CAD build for the part. Positions are in the model's coordinates, mm. Give positions to 0.01 mm unless a question says otherwise; leave off trailing zeros. Write each loop counter-clockwise with the first axis right and the second up, starting at its lowest first coordinate (ties: lowest second). Pieces come first, ordered by that corner, then holes. Notation, with made-up numbers: (-30.75, 14) - (21.25, 14) arc R17 ccw to (21.25, 39) - close; hole circle Ø3 at (51, 29.25). An arc over 180 degrees is marked (long way). Put each result on its own line as item: value. Start each with the question number.
1. Mould opens along X. For faces 1 (the flat face through (-34, 0, 33)), 2 (the cylindrical face through (-10.84, 98.6, 48.81)), 3 (the cylindrical face through (-10.189, 98.6, 45.882)) say: +X half, -X half, draft (parallel to the pull), parting line (faces both ways), or undercut.
2. Wall check: line 1 (Z direction, x = 0, y = 80.5); line 2 (X direction, y = 63, z = 24). Give the ranges that are in metal, low to high.
3. Drop flat-ended pins along their axis: pin 1 (1 mm diameter, centred on y = 99.5, z = 15, fed in from +X); pin 2 (6 mm diameter, centred on x = -35, y = 69.5, fed in from +Z); pin 3 (8 mm diameter, centred on y = 81, z = 32, fed in from +X). Give the stop position or say it passes through.
4. Cut at C-C on y = 52. List the corners of the cut face in (x, z).
5. Cut at B-B on x = 0. List the corners of the cut face in (y, z).
6. Cut at A-A on z = 0. List the corners of the cut face in (x, y), and give its area (3 significant figures).
from build123d import *

# Parameters (mm, degrees)
EXTRUDE_1_OUTLINE_R      = 50
EXTRUDE_1_OUTLINE_R_2    = 47
EXTRUDE_1_DEPTH          = 200
CUT_EXTRUDE_1_DEPTH      = 213.132034356
CUT_EXTRUDE_1_DEPTH_BACK = 213.132034356
SKETCH_2_R               = 62.5


# Read off the part's stored shape, not the designer's step: Вытянуть-Тонкостенный1
with BuildPart() as part:
    # Вытянуть-Тонкостенный1 outline → Вытянуть-Тонкостенный1 (new body)
    with BuildSketch(Plane(origin=(0, 0, 0), x_dir=(1, 0, 0), z_dir=(0, 1, 0))):
        Circle(EXTRUDE_1_OUTLINE_R)
        Circle(EXTRUDE_1_OUTLINE_R_2, mode=Mode.SUBTRACT)
    extrude(amount=EXTRUDE_1_DEPTH)

    # Эскиз2 → Вырез-Вытянуть1 (cut, two sides: drawn at the far end of the back side and taken through both)
    with BuildSketch(Plane(origin=(0, 0, 0), x_dir=(1, 0, 0), z_dir=(0, -0.819152044288991, -0.5735764363510473)).offset(-CUT_EXTRUDE_1_DEPTH_BACK)):
        with Locations((0, -180)):
            Circle(SKETCH_2_R)
    extrude(amount=CUT_EXTRUDE_1_DEPTH + CUT_EXTRUDE_1_DEPTH_BACK, mode=Mode.SUBTRACT)


solid = part.part
Report:
1. face 1: draft
1. face 2: parting line
1. face 3: undercut
2. line 1: z = -50 to -47, 47 to 50
2. line 2: x = -43.86 to -40.41, 40.41 to 43.86
3. pin 1: stops at x = 47.85
3. pin 2: stops at z = 38.42
3. pin 3: stops at x = 41.42
4. outline: circle Ø100 at (0, 0); hole circle Ø94 at (0, 0)
5. outline: (0, -50) - (133.45, -50) - (137.73, -47) - (0, -47) - close; (0, 47) - (200, 47) - (200, 50) - (0, 50) - close
6. outline: (-50, 0) - (-47, 0) - (-47, 200) - (-50, 200) - close; (47, 0) - (50, 0) - (50, 200) - (47, 200) - close
6. area: 1,200 mm²
